Geometry check sheet. Reference: the model listing, model coordinates, mm. Face numbers are marked on the shaded views. Round coordinates to 2 decimals unless told otherwise and drop trailing zeros. Loops run counter-clockwise (first coordinate to the right, second up) from the corner with the lowest first, then second, coordinate; pieces in that order, holes last. Notation, with made-up numbers: M 16,41 L 54,41 A12 cw 54,63 Z; hole C 85,-32.75 d1. An arc over 180 degrees is marked long. Answer in a Markdown table with one row per item. Add a question column.
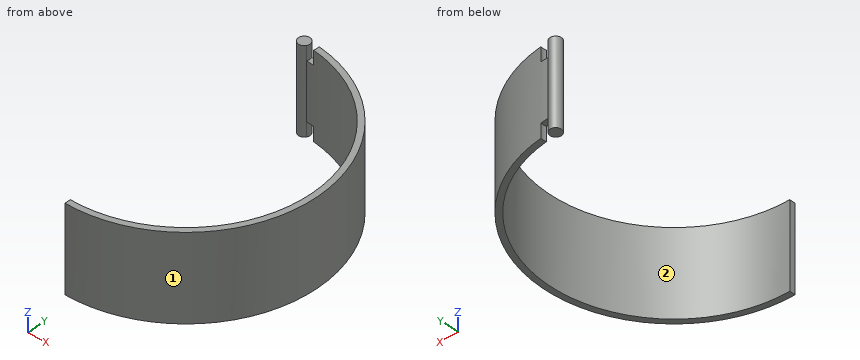
```python
from build123d import *

# Parameters (mm, degrees)
SKETCH_1_R          = 1
EXTRUDE_1_DEPTH     = 15
EXTRUDE_2_DEPTH     = 15
CUT_EXTRUDE_1_DEPTH = 2.5
CUT_EXTRUDE_2_DEPTH = 2.5


with BuildPart() as part:
    # ｽｹｯﾁ1 → ﾎﾞｽ - 押し出し1 (new body)
    with BuildSketch(Plane.XY):
        Circle(SKETCH_1_R)
    extrude(amount=EXTRUDE_1_DEPTH)

    # ｽｹｯﾁ2 → ﾎﾞｽ - 押し出し2 (add)
    with BuildSketch(Plane.XY.offset(15)):
        with BuildLine():
            Line((0, -44.5), (0, -45.5))
            ThreePointArc((0, -45.5), (23, -22.5), (0, 0.5))
            Line((0, 0.5), (0, -0.5))
            ThreePointArc((0, -0.5), (22, -22.5), (0, -44.5))
        make_face()
    extrude(amount=-EXTRUDE_2_DEPTH)

    # ｽｹｯﾁ3 → ｶｯﾄ - 押し出し1 (cut)
    with BuildSketch(Plane.XY.offset(15)):
        with BuildLine():
            ThreePointArc((0.875436399, 0.483333333), (0.999814775, -0.019246198), (0.856186636, -0.516666667))
            ThreePointArc((0.856186636, -0.516666667), (1.51206294, -0.552023654), (2.166591434, -0.606944444))
            ThreePointArc((2.166591434, -0.606944444), (2.247324467, -0.109693843), (2.215402295, 0.393055556))
            ThreePointArc((2.215402295, 0.393055556), (1.546078419, 0.44797685), (0.875436399, 0.483333333))
        make_face()
    extrude(amount=-CUT_EXTRUDE_1_DEPTH, mode=Mode.SUBTRACT)

    # ｽｹｯﾁ4 → ｶｯﾄ - 押し出し2 (cut)
    with BuildSketch(Plane(origin=(0, 0, 0), x_dir=(-1, 0, 0), z_dir=(0, 0, -1))):
        with BuildLine():
            ThreePointArc((-0.875436399, 0.483333333), (-0.999814775, -0.019246198), (-0.856186636, -0.516666667))
            ThreePointArc((-0.856186636, -0.516666667), (-1.51206294, -0.552023654), (-2.166591434, -0.606944444))
            ThreePointArc((-2.166591434, -0.606944444), (-2.247324467, -0.109693843), (-2.215402295, 0.393055556))
            ThreePointArc((-2.215402295, 0.393055556), (-1.546078419, 0.44797685), (-0.875436399, 0.483333333))
        make_face()
    extrude(amount=-CUT_EXTRUDE_2_DEPTH, mode=Mode.SUBTRACT)


solid = part.part
```
1) Cross-section at C-C, the plane y = -22.5. Record the boundary of the cut face in (x, z).
2) Cross-section at A-A, the plane x = 18. Record the boundary of the cut face in (y, z), plus the area to 3 significant figures.
3) Thickness scan on L1, parallel to X at y = -23, z = 8.5; L2, parallel to Y at x = 7.75, z = 2; L3, parallel to Y at x = 17.25, z = 13.25. Record the ranges inside material, lowest first. Write a range as [from, to].
4) Cross-section at B-B, the plane z = 14. Record the boundary of the cut face in (x, y).
5) Go/stop test with flat-tipped pins: pin 1 (8 mm diameter, centred on y = -39, z = 2.5, fed in from +X); pin 2 (0.5 mm diameter, centred on y = -45, z = 8, fed in from -X); pin 3 (0.9 mm diameter, centred on x = 1.5, y = 0, fed in from +Z). Record where each tip stops, or that it passes through.
6) Draft check along Y on the marked faces 1 and 2. Enter one of: +Y half, -Y half, draft (parallel to the pull), parting line (faces both ways), or undercut.
7) Cross-section at D-D, the plane x = 3.25. Record the boundary of the cut face in (y, z).
Worked answers:
| question | item | result |
|---|---|---|
| 1 | outline | M 22,0 L 23,0 L 23,15 L 22,15 Z |
| 2 | outline | M -36.82,0 L -35.15,0 L -35.15,15 L -36.82,15 Z; M -9.85,0 L -8.18,0 L -8.18,15 L -9.85,15 Z |
| 2 | area | 50.1 mm2 |
| 3 | L1 | x = [21.99, 22.99] |
| 3 | L2 | y = [-44.15, -43.09], [-1.91, -0.85] |
| 3 | L3 | y = [-37.71, -36.15], [-8.85, -7.29] |
| 4 | outline | C 0,0 d2; M 0,-45.5 A23 ccw 2.22,0.39 A2.25 cw 2.17,-0.61 A22 cw 0,-44.5 Z |
| 5 | pin 1 | stops at x = 19.31 |
| 5 | pin 2 | stops at x = 0 |
| 5 | pin 3 | stops at z = 12.5 |
| 6 | face 1 | parting line |
| 6 | face 2 | undercut |
| 7 | outline | M -45.27,0 L -44.26,0 L -44.26,15 L -45.27,15 Z; M -0.74,0 L 0.27,0 L 0.27,15 L -0.74,15 Z |
